The listing builds one solid part. Answer for the finished solid, in the listing's coordinates (mm). A direction names the side the tool comes from. Round coordinates to 2 decimals unless told otherwise and drop trailing zeros. Order: outer loops, then holes, each group sorted by start corner. A loop starts at its lowest first (then second) coordinate and runs counter-clockwise, first axis right, second up. Notation, with made-up numbers: (-6, 18.25) -> (33, 18.25) arc R22 ccw to (33, 49.25) -> close; hole circle Ø1 at (-32.5, 86). An arc over 180 degrees is marked (long way). Answer in a Markdown table with one row per item. Add a question column.
```python
from build123d import *

# Parameters (mm, degrees)
SKETCH_1_W          = 240
SKETCH_1_H          = 70
EXTRUDE_1_DEPTH     = 3
SKETCH_4_W          = 156
SKETCH_4_H          = 65
EXTRUDE_3_DEPTH     = 3
SKETCH_5_R          = 1.5
CUT_EXTRUDE_1_DEPTH = 20
FILLET_1_R          = 10
FILLET_2_R          = 10
SKETCH_7_W          = 130
SKETCH_7_H          = 35
CUT_EXTRUDE_2_DEPTH = 3
SKETCH_8_W          = 130
SKETCH_8_H          = 20
CUT_EXTRUDE_3_DEPTH = 3
CHAMFER_1_SIZE      = 0.5
CHAMFER_2_SIZE      = 0.5


with BuildPart() as part:
    # 草图1 → 凸台-拉伸1 (new body)
    with BuildSketch(Plane(origin=(0, 0, 0), x_dir=(0, 0, -1), z_dir=(1, 0, 0))):
        with Locations((0, 10)):
            Rectangle(SKETCH_1_W, SKETCH_1_H)
    extrude(amount=EXTRUDE_1_DEPTH)

    # 草图4 → 凸台-拉伸3 (add)
    with BuildSketch(Plane(origin=(3, 0, 0), x_dir=(0, 0, -1), z_dir=(1, 0, 0))):
        with Locations((0, 12.5)):
            Rectangle(SKETCH_4_W, SKETCH_4_H)
    extrude(amount=EXTRUDE_3_DEPTH)

    # 草图5 → 切除-拉伸1 (cut)
    with BuildSketch(Plane.ZY):
        with Locations((113, 25)):
            Circle(SKETCH_5_R)
        with Locations((113, -5)):
            Circle(SKETCH_5_R)
        with Locations(Location((-113, -5, 0), (0, 0, 180))):
            Circle(SKETCH_5_R)
        with Locations(Location((-113, 25, 0), (0, 0, 180))):
            Circle(SKETCH_5_R)
    extrude(amount=-CUT_EXTRUDE_1_DEPTH, mode=Mode.SUBTRACT)

    # 圆角1
    fillet_1_edges = [part.edges().sort_by_distance(p)[0] for p in [
        (1.5, -25, -120),
        (1.5, -25, 120),
    ]]
    fillet(fillet_1_edges, radius=FILLET_1_R)

    # 圆角2
    fillet_2_edges = [part.edges().sort_by_distance(p)[0] for p in [
        (4.5, -20, 78),
        (4.5, -20, -78),
    ]]
    fillet(fillet_2_edges, radius=FILLET_2_R)

    # 草图7 → 切除-拉伸2 (cut)
    with BuildSketch(Plane.ZY):
        with Locations((0, 27.5)):
            Rectangle(SKETCH_7_W, SKETCH_7_H)
    extrude(amount=-CUT_EXTRUDE_2_DEPTH, mode=Mode.SUBTRACT)

    # 草图8 → 切除-拉伸3 (cut)
    with BuildSketch(Plane.ZY.offset(-3)):
        with Locations((0, 35)):
            Rectangle(SKETCH_8_W, SKETCH_8_H)
    extrude(amount=-CUT_EXTRUDE_3_DEPTH, mode=Mode.SUBTRACT)

    # 倒角1
    chamfer_1_edges = [part.edges().sort_by_distance(p)[0] for p in [
        (0, 45, -92.5),
        (0, 45, 92.5),
    ]]
    chamfer(chamfer_1_edges, length=CHAMFER_1_SIZE)

    # 倒角2
    chamfer_2_edges = [part.edges().sort_by_distance(p)[0] for p in [
        (0, 27.25, 65),
        (0, 10, 0),
        (0, 27.25, -65),
    ]]
    chamfer(chamfer_2_edges, length=CHAMFER_2_SIZE)


solid = part.part
```
Item 1: The part is cut by section A-A, the plane x = 4.75. Give the vertices of the cut face in (y, z), and give its area (3 significant figures).
Item 2: A tool of negligible diameter and unlimited length cuts with its end or side. For faces 1 (the face through (4.52, -16.99, -75.15)), 2 (the face through (4.52, -16.99, 75.15)), 3 (the face through (3, 18, -1)), from which of +Z, -Z, +X, -X, +Y, -Y can it reach the whole face along a straight path? Write none if from no direction.
Item 3: Flat-ended cylindrical pins translate along their axes: P1, Ø2.5, axis at x = 4.5, z = 6, coming from the +Y side; P2, Ø16.5, axis at y = 18, z = -11.5, coming from the -X side; P3, Ø1.5, axis at x = 5.5, y = 10.5, coming from the -Z side. Find the tip coordinate at first contact, or state that the pin passes through.
Item 4: The part is cut by section C-C, the plane z = -85. Give the vertices of the cut face in (x, y), and give its area (3 significant figures).
Item 5: Find the intervals of material crossed by probe 1 along Z at (x, y) = (5.75, 36.5); probe 2 along Z at (x, y) = (2.5, 13.5); probe 3 along Y at (x, z) = (2.45, -113), in increasing order. Write a range as [from, to].
Item 6: The part is cut by section B-B, the plane y = 15. Give the vertices of the cut face in (x, z).
Resolved:
| question | item | result |
|---|---|---|
| 1 | outline | (-20, -68) arc R10 ccw to (-10, -78) -> (45, -78) -> (45, -65) -> (25, -65) -> (25, 65) -> (45, 65) -> (45, 78) -> (-10, 78) arc R10 ccw to (-20, 68) -> close |
| 1 | area | 7,500 mm2 |
| 2 | face 1 | -Z, +X, -Y |
| 2 | face 2 | +Z, +X, -Y |
| 2 | face 3 | -X, +Y |
| 3 | P1 | y = 25 |
| 3 | P2 | x = 0.25 |
| 3 | P3 | z = -78 |
| 4 | outline | (0, -25) -> (3, -25) -> (3, 45) -> (0.5, 45) -> (0, 44.5) -> close |
| 4 | area | 210 mm2 |
| 5 | probe 1 | [-78, -65], [65, 78] |
| 5 | probe 2 | [-120, -65], [65, 120] |
| 5 | probe 3 | [-24.54, -6.5], [-3.5, 23.5], [26.5, 45] |
| 6 | outline | (0, -120) -> (3, -120) -> (3, -78) -> (6, -78) -> (6, 78) -> (3, 78) -> (3, 120) -> (0, 120) -> (0, 65.5) -> (0.5, 65) -> (3, 65) -> (3, -65) -> (0.5, -65) -> (0, -65.5) -> close |
